```python
from build123d import *

# Parameters (mm, degrees)
SKETCH1_W                                            = 40
SKETCH1_H                                            = 30
BOSS_EXTRUDE1_DEPTH                                  = 10
SKETCH2_W                                            = 15
SKETCH2_H                                            = 15
CUT_EXTRUDE1_DEPTH                                   = 27.925824036
CBORE_FOR_M2_5_SLOTTED_CHEESE_HEAD_SCREW_D           = 2.9
CBORE_FOR_M2_5_SLOTTED_CHEESE_HEAD_SCREW_DEPTH       = 12.5
CBORE_FOR_M2_5_SLOTTED_CHEESE_HEAD_SCREW_CBORE_D     = 5
CBORE_FOR_M2_5_SLOTTED_CHEESE_HEAD_SCREW_CBORE_DEPTH = 2.9
M4_TAPPED_HOLE1_D                                    = 3.3
M4_TAPPED_HOLE1_DEPTH                                = 5
M4_TAPPED_HOLE1_TIP                                  = 0.991420021
FILLET1_R                                            = 1
CHAMFER1_SIZE                                        = 1
CHAMFER2_SIZE                                        = 1
M4_TAPPED_HOLE2_D                                    = 3.3


with BuildPart() as part:
    # Sketch1 → Boss-Extrude1 (new body)
    with BuildSketch(Plane.XY):
        Rectangle(SKETCH1_W, SKETCH1_H)
    extrude(amount=BOSS_EXTRUDE1_DEPTH)

    # Sketch2 → Cut-Extrude1 (cut, through all)
    with BuildSketch(Plane.XY.offset(10)):
        with Locations((0, -7.5)):
            Rectangle(SKETCH2_W, SKETCH2_H)
    extrude(amount=-CUT_EXTRUDE1_DEPTH, mode=Mode.SUBTRACT)

    # CBORE for M2.5 Slotted cheese head screws2
    with Locations(Plane.ZY.offset(20)):
        with Locations((5, -2.5), (5, -12)):
            cbore_for_m2_5_slotted_cheese_head_screw = CounterBoreHole(CBORE_FOR_M2_5_SLOTTED_CHEESE_HEAD_SCREW_D / 2, CBORE_FOR_M2_5_SLOTTED_CHEESE_HEAD_SCREW_CBORE_D / 2, CBORE_FOR_M2_5_SLOTTED_CHEESE_HEAD_SCREW_CBORE_DEPTH, depth=CBORE_FOR_M2_5_SLOTTED_CHEESE_HEAD_SCREW_DEPTH)

    # Mirror1: CBORE for M2.5 Slotted cheese head screws2 across plane
    add(cbore_for_m2_5_slotted_cheese_head_screw.mirror(Plane(origin=(0, 0, 0), x_dir=(0, 0, 1), z_dir=(1, 0, 0))), mode=Mode.SUBTRACT)

    # M4 Tapped Hole1
    with Locations(Plane(origin=(0, 0, 0), x_dir=(-1, 0, 0), z_dir=(0, 0, -1))):
        with Locations((-13.75, -7), (-13.75, 11), (13.75, 11), (13.75, -7)):
            Hole(M4_TAPPED_HOLE1_D / 2, depth=M4_TAPPED_HOLE1_DEPTH)
            with Locations((0, 0, -(M4_TAPPED_HOLE1_DEPTH + M4_TAPPED_HOLE1_TIP / 2))):  # 118° drill point
                Cone(0, M4_TAPPED_HOLE1_D / 2, M4_TAPPED_HOLE1_TIP, mode=Mode.SUBTRACT)

    # Fillet1
    fillet1_edges = [part.edges().sort_by_distance(p)[0] for p in [
        (7.5, 0, 5),
        (-7.5, 0, 5),
    ]]
    fillet(fillet1_edges, radius=FILLET1_R)

    # Chamfer1
    chamfer1_edges = [part.edges().sort_by_distance(p)[0] for p in [
        (7.5, -15, 5),
        (-7.5, -15, 5),
    ]]
    chamfer(chamfer1_edges, length=CHAMFER1_SIZE)

    # Chamfer2
    chamfer2_edges = [part.edges().sort_by_distance(p)[0] for p in [
        (7.5, -7.5, 0),
        (-7.5, -7.5, 0),
        (7.207106781, -0.292893219, 0),
        (-7.207106781, -0.292893219, 0),
        (0, 0, 0),
    ]]
    chamfer(chamfer2_edges, length=CHAMFER2_SIZE)

    # M4 Tapped Hole2 (through all)
    with Locations(Plane(origin=(0, 15, 0), x_dir=(1, 0, 0), z_dir=(0, 1, 0))):
        with Locations((0, -5)):
            Hole(M4_TAPPED_HOLE2_D / 2)


solid = part.part
```
Geometry: final body of the model. Coordinates: model frame, mm. A direction names the side the tool comes from. Round coordinates to 2 decimals unless told otherwise and drop trailing zeros. Write each loop counter-clockwise with the first axis right and the second up, starting at its lowest first coordinate (ties: lowest second). Pieces come first, ordered by that corner, then holes. Notation, with made-up numbers: (33.25, 15) -> (58.25, 15) arc R25 ccw to (58.25, 46) -> close; hole circle Ø2 at (79, -24). An arc over 180 degrees is marked (long way). Return JSON: item names as keys, results as strings.
Q1. Set-up query: faces 1 (the flat face through (-17.1, -14, 5)), 2 (the cylindrical face through (-12.226, 10.368, 2.535)), 3 (the flat face through (8, -14.5, 5.1)), 4 (the flat face through (14, -15, 5)). Return all of +Z, -Z, +X, -X, +Y, -Y with unobstructed straight access to the full face (end or side cutting, diameter ignored); none if empty.
From the geometry:
{"face 1": "-X", "face 2": "-Z", "face 3": "+Z, -Z, -Y", "face 4": "+Z, -Z, +X, -X, -Y"}
Q2. Ray query, line 1 (X direction, y = 11, z = 2.45); line 2 (Y direction, x = -13.75, z = 2.2); line 3 (Y direction, x = 12, z = 5). Return the intervals inside material, ascending.
From the geometry:
{"line 1": "-20 to -15.4, -12.1 to 12.1, 15.4 to 20", "line 2": "-15 to -8.65, -5.35 to 9.35, 12.65 to 15", "line 3": "-15 to -13.45, -10.55 to -3.95, -1.05 to 15"}
Q3. First-contact query: pin 1 Ø4 at (y, z) = (-12, 5) entering from -X; pin 2 Ø2 at (x, y) = (-13.75, -7) entering from -Z. Flat tips, straight axial feed; report the tip coordinate or a pass-through.
From the geometry:
{"pin 1": "x = -17.1", "pin 2": "z = 5.39"}
Q4. Section B-B on x = 0. Return the cut outline in (y, z), and give its area (3 significant figures).
From the geometry:
{"outline": "(0, 1) -> (1, 0) -> (15, 0) -> (15, 3.35) -> (0, 3.35) -> close; (0, 6.65) -> (15, 6.65) -> (15, 10) -> (0, 10) -> close", "area": "100 mm2"}
Q5. Mould query, pull axis Z, two halves, no side actions, for faces 5 (the cylindrical face through (-7.215, -0.301, 5.437)), 6 (the conical face through (-7.466, -0.012, 0.618)), 7 (the cylindrical face through (18.57, -14.22, 6.15)). Classes: +Z half, -Z half, draft (parallel to the pull), parting line (faces both ways), or undercut.
From the geometry:
{"face 5": "draft", "face 6": "-Z half", "face 7": "undercut"}
Q6. Section C-C on x = 10. Return the cut outline in (y, z).
From the geometry:
{"outline": "(-15, 0) -> (15, 0) -> (15, 10) -> (-15, 10) -> close; hole circle Ø2.9 at (-12, 5); hole circle Ø2.9 at (-2.5, 5)"}
Q7. Section D-D on z = 4.5. Give the number of separate pieces and of enclosed holes in the cut face, and give its area (3 significant figures).
From the geometry:
{"separate pieces": "6", "enclosed holes": "4", "area": "732 mm2"}
Q8. Section A-A on y = -2.5. Return the cut outline in (x, z), and give its area (3 significant figures).
From the geometry:
{"outline": "(-20, 0) -> (-8.5, 0) -> (-7.5, 1) -> (-7.5, 3.55) -> (-17.1, 3.55) -> (-17.1, 2.5) -> (-20, 2.5) -> close; (-20, 7.5) -> (-17.1, 7.5) -> (-17.1, 6.45) -> (-7.5, 6.45) -> (-7.5, 10) -> (-20, 10) -> close; (7.5, 1) -> (8.5, 0) -> (20, 0) -> (20, 2.5) -> (17.1, 2.5) -> (17.1, 3.55) -> (7.5, 3.55) -> close; (7.5, 6.45) -> (17.1, 6.45) -> (17.1, 7.5) -> (20, 7.5) -> (20, 10) -> (7.5, 10) -> close", "area": "164 mm2"}
